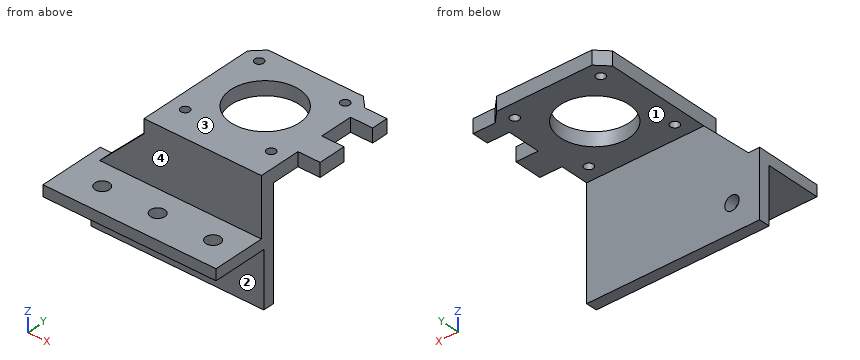
```python
from build123d import *

# Parameters (mm, degrees)
SKICA1_W                 = 62.391596743
SKICA1_H                 = 24
P_IDAT_VYSUNUT_M1_DEPTH  = 4
SKICA2_W                 = 42.3
SKICA2_H                 = 5
P_IDAT_VYSUNUT_M2_DEPTH  = 16
SKICA3_R                 = 1.6
SKICA3_R_2               = 12.36434098
P_IDAT_VYSUNUT_M5_DEPTH  = 5
ZKOSEN_1_SIZE            = 16
SKICA4_R                 = 2.6
ODEBRAT_VYSUNUT_M1_DEPTH = 4
SKICA5_W                 = 62.391596743
SKICA5_H                 = 4
P_IDAT_VYSUNUT_M6_DEPTH  = 20
SKICA6_R                 = 2.6
ODEBRAT_VYSUNUT_M2_DEPTH = 4
SKICA7_W                 = 5
SKICA7_H                 = 6
SKICA7_H_2               = 10
P_IDAT_VYSUNUT_M7_DEPTH  = 8


with BuildPart() as part:
    # Skica1 → Přidat vysunutím1 (new body)
    with BuildSketch(Plane.XY):
        with Locations((-71.195798372, -0.971059771)):
            Rectangle(SKICA1_W, SKICA1_H)
    extrude(amount=P_IDAT_VYSUNUT_M1_DEPTH)

    # Skica2 → Přidat vysunutím2 (add)
    with BuildSketch(Plane.XY.offset(4)):
        with Locations((-61.15, 8.528940229)):
            Rectangle(SKICA2_W, SKICA2_H)
    extrude(amount=P_IDAT_VYSUNUT_M2_DEPTH)

    # Skica3 → Přidat vysunutím5 (add)
    with BuildSketch(Plane.XY.offset(20)):
        Polygon((-40, 6.028940229), (-82.3, 6.028940229), (-82.3, 49.328940229), (-78.3, 53.328940229), (-44, 53.328940229), (-40, 49.328940229), align=None)
        with Locations((-45.65, 47.678940229)):
            Circle(SKICA3_R, mode=Mode.SUBTRACT)
        with Locations((-76.65, 47.678940229)):
            Circle(SKICA3_R, mode=Mode.SUBTRACT)
        with Locations((-76.65, 16.678940229)):
            Circle(SKICA3_R, mode=Mode.SUBTRACT)
        with Locations((-45.65, 16.678940229)):
            Circle(SKICA3_R, mode=Mode.SUBTRACT)
        with Locations((-61.15, 32.178940229)):
            Circle(SKICA3_R_2, mode=Mode.SUBTRACT)
    extrude(amount=P_IDAT_VYSUNUT_M5_DEPTH)

    # Zkosení1
    zkosen_1_edges = [part.edges().sort_by_distance(p)[0] for p in [
        (-82.3, 8.528940229, 4),
    ]]
    chamfer(zkosen_1_edges, length=ZKOSEN_1_SIZE)

    # Skica4 → Odebrat vysunutím1 (cut)
    with BuildSketch(Plane.XY.offset(4)):
        with Locations((-89.655606689, -2.971059771)):
            Circle(SKICA4_R)
        with Locations((-69.655606689, -2.971059771)):
            Circle(SKICA4_R)
        with Locations((-49.655606689, -2.971059771)):
            Circle(SKICA4_R)
    extrude(amount=-ODEBRAT_VYSUNUT_M1_DEPTH, mode=Mode.SUBTRACT)

    # Skica5 → Přidat vysunutím6 (add)
    with BuildSketch(Plane(origin=(0, 0, 0), x_dir=(-1, 0, 0), z_dir=(0, 0, -1))):
        with Locations((71.195798372, 9.028940229)):
            Rectangle(SKICA5_W, SKICA5_H)
    extrude(amount=P_IDAT_VYSUNUT_M6_DEPTH)

    # Skica6 → Odebrat vysunutím2 (cut)
    with BuildSketch(Plane(origin=(0, 11.028940229, 0), x_dir=(1, 0, 0), z_dir=(0, 1, 0))):
        with Locations(Location((-92.391596743, 10, 0), (0, 0, 270))):
            Circle(SKICA6_R)
    extrude(amount=-ODEBRAT_VYSUNUT_M2_DEPTH, mode=Mode.SUBTRACT)

    # Skica7 → Přidat vysunutím7 (add)
    with BuildSketch(Plane(origin=(-40, 0, 0), x_dir=(0, 0, -1), z_dir=(1, 0, 0))):
        with Locations((-22.5, 46.328940229)):
            Rectangle(SKICA7_W, SKICA7_H)
        with Locations((-22.5, 26.328940229)):
            Rectangle(SKICA7_W, SKICA7_H_2)
    extrude(amount=P_IDAT_VYSUNUT_M7_DEPTH)


solid = part.part
```
The model under review builds one solid part; all positions refer to its coordinate system, in mm. Face numbers are marked on the shaded views. A direction names the side the tool comes from. Round coordinates to 2 decimals unless told otherwise and drop trailing zeros. Order: outer loops, then holes, each group sorted by start corner. A loop starts at its lowest first (then second) coordinate and runs counter-clockwise, first axis right, second up.
Item 1: Add section D-D, the plane x = -60.5. State the section outline as (y, z) points, and give its area (3 significant figures).
Working result:
outline: (-12.97, 0) - (7.03, 0) - (7.03, -20) - (11.03, -20) - (11.03, 20) - (19.83, 20) - (19.83, 25) - (6.03, 25) - (6.03, 4) - (-12.97, 4) - close; (44.53, 20) - (53.33, 20) - (53.33, 25) - (44.53, 25) - close
area: 369 mm2
Item 2: Add section A-A, the plane x = -45.65. State the section outline as (y, z) points.
Working result:
outline: (-12.97, 0) - (7.03, 0) - (7.03, -20) - (11.03, -20) - (11.03, 20) - (15.08, 20) - (15.08, 25) - (6.03, 25) - (6.03, 4) - (-12.97, 4) - close; (18.28, 20) - (46.08, 20) - (46.08, 25) - (18.28, 25) - close; (49.28, 20) - (53.33, 20) - (53.33, 25) - (49.28, 25) - close
Item 3: Machinability: for the marked faces 1, 2, 3 and 4, which of the approach directions +Z, -Z, +X, -X, +Y, -Y give a long, thin tool a straight path to every point of the face, cutting with its end or side? Answer none if there is none.
Working result:
face 1: -Z, +X, -X, +Y
face 2: -Z, +X, -X, -Y
face 3: +Z, +X, -X, +Y, -Y
face 4: +Z, +X, -X, -Y
Item 4: To check wall thickness, follow probe 1 along Y at (x, z) = (-76, 22); probe 2 along Y at (x, z) = (-87, -18); probe 3 along Y at (x, z) = (-96, 2). State the ranges of each line that lie inside material, in increasing order.
Working result:
probe 1: y = 6.03 to 15.22, 18.14 to 46.22, 49.14 to 53.33
probe 2: y = 7.03 to 11.03
probe 3: y = -12.97 to 11.03
Item 5: For pin 1 (5.5 mm diameter, centred on y = 37.5, z = 22.5, fed in from +X); pin 2 (3 mm diameter, centred on x = -45.65, y = 47.68, fed in from +Z); pin 3 (10 mm diameter, centred on x = -62, z = -11, fed in from -Y); pin 4 (1.5 mm diameter, centred on x = -40, y = 38, fed in from -Z), all flat-tipped, find the tip position at first contact; note any pin that passes through.
Working result:
pin 1: stops at x = -40
pin 2: passes through
pin 3: stops at y = 7.03
pin 4: stops at z = 20
Item 6: Add section B-B, the plane z = -10. State the section outline as (x, y) points, and give its area (3 significant figures).
Working result:
outline: (-102.39, 7.03) - (-94.99, 7.03) - (-94.99, 11.03) - (-102.39, 11.03) - close; (-89.79, 7.03) - (-40, 7.03) - (-40, 11.03) - (-89.79, 11.03) - close
area: 229 mm2
Item 7: Add section C-C, the plane y = 37.5. State the section outline as (x, z) points, and give its area (3 significant figures).
Working result:
outline: (-82.3, 20) - (-72.31, 20) - (-72.31, 25) - (-82.3, 25) - close; (-49.99, 20) - (-40, 20) - (-40, 25) - (-49.99, 25) - close
area: 99.9 mm2
